The model under review builds one solid part; all positions refer to its coordinate system, in mm. Face numbers are marked on the shaded views. A direction names the side the tool comes from. Round coordinates to 2 decimals unless told otherwise and drop trailing zeros. Write each loop counter-clockwise with the first axis right and the second up, starting at its lowest first coordinate (ties: lowest second). Pieces come first, ordered by that corner, then holes. Notation, with made-up numbers: (9, 34) - (16, 34) arc R20 ccw to (16, 69) - close; hole circle Ø7 at (-36, 87.5). An arc over 180 degrees is marked (long way). Return JSON: item names as keys, results as strings.
from build123d import *

# Parameters (mm, degrees)
BOSS_EXTRUDE1_DEPTH = 5
SKETCH2_W           = 8
SKETCH2_H           = 7
BOSS_EXTRUDE2_DEPTH = 10
SKETCH3_W           = 42
SKETCH3_H           = 8
BOSS_EXTRUDE3_DEPTH = 40


with BuildPart() as part:
    # Sketch1 → Boss-Extrude1 (new body)
    with BuildSketch(Plane.XY):
        Polygon((-17.516022594, -16.039535536), (24.483977406, -16.039535536), (24.483977406, 13.960464464), (16.483977406, 13.960464464), (16.483977406, 3.460464464), (-9.516022594, 3.460464464), (-9.516022594, 13.960464464), (-17.516022594, 13.960464464), align=None)
    extrude(amount=BOSS_EXTRUDE1_DEPTH)

    # Sketch2 → Boss-Extrude2 (add)
    with BuildSketch(Plane(origin=(0, 0, 0), x_dir=(-1, 0, 0), z_dir=(0, 0, -1))):
        with Locations((-20.483977406, -0.539535536)):
            Rectangle(SKETCH2_W, SKETCH2_H)
        with Locations((13.516022594, -0.539535536)):
            Rectangle(SKETCH2_W, SKETCH2_H)
    extrude(amount=BOSS_EXTRUDE2_DEPTH)

    # Sketch3 → Boss-Extrude3 (add)
    with BuildSketch(Plane.XY.offset(5)):
        with Locations((3.483977406, -12.039535536)):
            Rectangle(SKETCH3_W, SKETCH3_H)
    extrude(amount=BOSS_EXTRUDE3_DEPTH)


solid = part.part
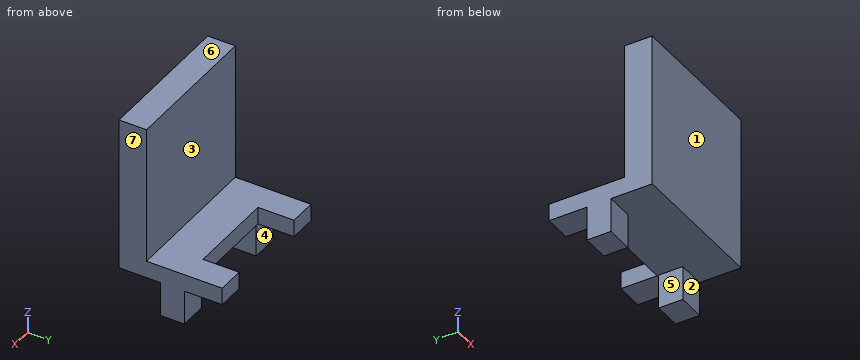
(1) Add section B-B (z = -1.5). Write out the cut boundary in (x, y).
Filled in:
{"outline": "(-17.52, -4.04) - (-9.52, -4.04) - (-9.52, 2.96) - (-17.52, 2.96) - close; (16.48, -4.04) - (24.48, -4.04) - (24.48, 2.96) - (16.48, 2.96) - close"}
(2) Mouldability with a two-part tool opening along X and no side actions: class the marked faces 5, 6 and 7 as released by +X, released by -X, zero draft, split by the parting line, or undercut.
Filled in:
{"face 5": "undercut", "face 6": "zero draft", "face 7": "released by +X"}
(3) Add section C-C (y = -1). Write out the cut boundary in (x, z), plus the area to 3 significant figures.
Filled in:
{"outline": "(-17.52, -10) - (-9.52, -10) - (-9.52, 0) - (16.48, 0) - (16.48, -10) - (24.48, -10) - (24.48, 5) - (-17.52, 5) - close", "area": "370 mm2"}
(4) Wall thickness on line 1 (X direction, y = 7, z = 4); line 2 (Y direction, x = 0.5, z = 34); line 3 (Y direction, x = 17.5, z = -6.5): over which ranges is each line inside the solid? List them lowest first.
Filled in:
{"line 1": "x = -17.52 to -9.52, 16.48 to 24.48", "line 2": "y = -16.04 to -8.04", "line 3": "y = -4.04 to 2.96"}
(5) Add section A-A (y = 7). Write out the cut boundary in (x, z).
Filled in:
{"outline": "(-17.52, 0) - (-9.52, 0) - (-9.52, 5) - (-17.52, 5) - close; (16.48, 0) - (24.48, 0) - (24.48, 5) - (16.48, 5) - close"}
(6) Add section D-D (x = 11). Write out the cut boundary in (y, z).
Filled in:
{"outline": "(-16.04, 0) - (3.46, 0) - (3.46, 5) - (-8.04, 5) - (-8.04, 45) - (-16.04, 45) - close"}
(7) Clearance check with flat-ended pins moving along their axes: pin 1 Ø8 at (x, z) = (11, 10.5) entering from +Y; pin 2 Ø3 at (x, y) = (-1, -10) entering from -Z; pin 3 Ø2.5 at (x, z) = (-14, -7) entering from -Y. State where each tip first meets the part, or that it passes through.
Filled in:
{"pin 1": "stops at y = -8.04", "pin 2": "stops at z = 0", "pin 3": "stops at y = -4.04"}
(8) For the marked faces 1, 2, 3 and 4, list the 3-axis set-ups (+Z, -Z, +X, -X, +Y, -Y) from which the entire face can be reached by the end or side of a thin tool; tool diameter is ignored.
Filled in:
{"face 1": "+Z, -Z, +X, -X, -Y", "face 2": "-Z, +X, -X, -Y", "face 3": "+Z, +X, -X, +Y", "face 4": "-Z, +X, -X, +Y"}
